```python
from build123d import *

# Parameters (mm, degrees)
F1_DEPTH  = 50.8
F2_W      = 50.8
F2_H      = 50.8
F3_DEPTH  = 1016
F5_W      = 50.8
F5_H      = 50.8
F6_DEPTH  = 381
F9_DEPTH  = 1066.801
F11_W     = 50.8
F11_H     = 50.8
F12_DEPTH = 152.4


with BuildPart() as f1:
    # F0 (on Front) → F1 (new body)
    with BuildSketch(Plane.XZ):
        Polygon((685.8, 50.8), (-203.2, 50.8), (685.8, -838.2), align=None)
    extrude(amount=F1_DEPTH)

    # F2 (on face) → F3 (join)
    with BuildSketch(Plane(origin=(0, 0, 0), x_dir=(-1, 0, 0), z_dir=(0, 1, 0))):
        with Locations((-660.4, 25.4)):
            Rectangle(F2_W, F2_H)
    extrude(amount=F3_DEPTH)

    # F5 (on face) → F6 (join)
    with BuildSketch(Plane.YZ.offset(685.8)):
        with Locations((-25.4, 25.4)):
            Rectangle(F5_W, F5_H)
    extrude(amount=F6_DEPTH)

    # F8 (on face) → F9 (cut, through all)
    with BuildSketch(Plane.XZ.offset(50.8)):
        Polygon((635, -715.5579510314), (635, 0), (-80.5579510314, 0), align=None)
    extrude(amount=-F9_DEPTH, mode=Mode.SUBTRACT)

    # F11 (on face) → F12 (join)
    with BuildSketch(Plane(origin=(0, 0, 0), x_dir=(1, 0, 0), z_dir=(0, 0, -1))):
        with Locations((1041.4, 25.4)):
            Rectangle(F11_W, F11_H)
    extrude(amount=F12_DEPTH)

    # F13: F1 across plane


with BuildPart() as f1_1:
    add(f1.part)
    add(f1.part.mirror(Plane(origin=(660.4, 1016, 25.4), x_dir=(-1, 0, 0), z_dir=(0, 1, 0))))


solid = f1_1.part
```
Work out the finished part from the listing and answer in its coordinate system (mm). A direction names the side the tool comes from. Coordinates: 2 decimals unless noted, no trailing zeros. Write each loop counter-clockwise with the first axis right and the second up, starting at its lowest first coordinate (ties: lowest second). Pieces come first, ordered by that corner, then holes. Notation, with made-up numbers: (60, 4) - (88, 4) arc R25 cw to (88, 22) - close; hole circle Ø11 at (30, 35). An arc over 180 degrees is marked (long way). Answer as a JSON object with one key per item and string values.
Q1. Find section B-B (x = 28.5). Write down the section's boundary in (y, z).
Results list:
{"outline": "(-50.8, -180.9) - (0, -180.9) - (0, -109.06) - (-50.8, -109.06) - close; (-50.8, 0) - (0, 0) - (0, 50.8) - (-50.8, 50.8) - close; (2032, -180.9) - (2082.8, -180.9) - (2082.8, -109.06) - (2032, -109.06) - close; (2032, 0) - (2082.8, 0) - (2082.8, 50.8) - (2032, 50.8) - close"}
Q2. Find section D-D (y = 266). Write down the section's boundary in (x, z), plus the area to 3 significant figures.
Results list:
{"outline": "(635, 0) - (685.8, 0) - (685.8, 50.8) - (635, 50.8) - close", "area": "2,580 mm^2"}
Q3. Which of the six approach directions +Z, -Z, +X, -X, +Y, -Y give full straight-line access (tool end or side, diameter ignored) to faces 1 (the flat face through (849, -26, 0)), 2 (the flat face through (239, 2032, -326)), 3 (the flat face through (272.21, 2057.76, -352.77)), 4 (the flat face through (685.8, 1030, 25))?
Results list:
{"face 1": "-Z, +Y, -Y", "face 2": "-Z, -X", "face 3": "+Y, -Y", "face 4": "+Z, -Z, +X"}
Q4. Find section A-A (x = 983.5). Write down the section's boundary in (y, z), plus the area to 3 significant figures.
Results list:
{"outline": "(-50.8, 0) - (0, 0) - (0, 50.8) - (-50.8, 50.8) - close; (2032, 0) - (2082.8, 0) - (2082.8, 50.8) - (2032, 50.8) - close", "area": "5,160 mm^2"}
Q5. Consider L1, parallel to Z at x = 677, y = 1196.5; L2, parallel to X at y = 1486.5, z = 13. Determine where each line is inside the solid, lowest interval first. Write a range as from..to.
Results list:
{"L1": "z = 0..50.8", "L2": "x = 635..685.8"}
Q6. Given pin 1 Ø15 at (y, z) = (-23, -50) entering from -X; pin 2 Ø15 at (y, z) = (2057, -53.5) entering from -X; pin 3 Ø15 at (x, y) = (181.5, -26) entering from -Z, each flat-ended and moving along its own axis, determine where each tip first touches the part or whether it passes through.
Results list:
{"pin 1": "stops at x = -109.9", "pin 2": "stops at x = -106.4", "pin 3": "stops at z = -341.4"}
Q7. Find section C-C (z = -60). Write down the section's boundary in (x, y).
Results list:
{"outline": "(-92.4, -50.8) - (-20.56, -50.8) - (-20.56, 0) - (-92.4, 0) - close; (-92.4, 2032) - (-20.56, 2032) - (-20.56, 2082.8) - (-92.4, 2082.8) - close; (635, -50.8) - (685.8, -50.8) - (685.8, 0) - (635, 0) - close; (635, 2032) - (685.8, 2032) - (685.8, 2082.8) - (635, 2082.8) - close; (1016, -50.8) - (1066.8, -50.8) - (1066.8, 0) - (1016, 0) - close; (1016, 2032) - (1066.8, 2032) - (1066.8, 2082.8) - (1016, 2082.8) - close"}
Q8. For a pull along Y with two mould halves and no side action, classify faces 5 (the flat face through (239, 0, -326)), 6 (the flat face through (664, 1021, 50.8)) as pulls with the +Y half, pulls with the -Y half, needs draft (parallel to the pull), parting line crosses it, or undercut.
Results list:
{"face 5": "undercut", "face 6": "needs draft"}
